```python
from build123d import *

# Parameters (mm, degrees)
BOSS_EXTRUDE1_DEPTH = 9
BOSS_EXTRUDE2_DEPTH = 11
SKETCH4_W           = 15
SKETCH4_H           = 5
CUT_EXTRUDE1_DEPTH  = 3


with BuildPart() as part:
    # Sketch2 → Boss-Extrude1 (new body)
    with BuildSketch(Plane(origin=(0, 0, 0), x_dir=(1, 0, 0), z_dir=(0, 1, 0))):
        with BuildLine():
            ThreePointArc((-13.134406493, 3.867125393), (0, 3), (13.134406493, 3.867125393))
            Line((13.134406493, 3.867125393), (13.134406493, -3.867125393))
            ThreePointArc((13.134406493, -3.867125393), (0, -3), (-13.134406493, -3.867125393))
            Line((-13.134406493, -3.867125393), (-13.134406493, 3.867125393))
        make_face()
    extrude(amount=BOSS_EXTRUDE1_DEPTH)

    # Sketch3 → Boss-Extrude2 (add)
    with BuildSketch(Plane(origin=(0, 9, 0), x_dir=(1, 0, 0), z_dir=(0, 1, 0))):
        with BuildLine():
            Line((13.134406493, -3.867125393), (13.134406493, 3.867125393))
            ThreePointArc((13.134406493, 3.867125393), (0, 3), (-13.134406493, 3.867125393))
            Line((-13.134406493, 3.867125393), (-13.134406493, -3.867125393))
            ThreePointArc((-13.134406493, -3.867125393), (0, -3), (13.134406493, -3.867125393))
        make_face()
    extrude(amount=BOSS_EXTRUDE2_DEPTH)

    # Sketch4 → Cut-Extrude1 (cut)
    with BuildSketch(Plane.XZ):
        Rectangle(SKETCH4_W, SKETCH4_H)
    extrude(amount=-CUT_EXTRUDE1_DEPTH, mode=Mode.SUBTRACT)


solid = part.part
```
Can you work these out from the model? Positions are in its coordinate system, mm. A direction names the side the tool comes from. Coordinates: 2 decimals unless noted, no trailing zeros. Loops run counter-clockwise (first coordinate to the right, second up) from the corner with the lowest first, then second, coordinate; pieces in that order, holes last. Notation, with made-up numbers: (82, -22) -> (93, -22) arc R16 ccw to (93, -5) -> close; hole circle Ø3 at (-25.75, 81). An arc over 180 degrees is marked (long way). Put each result on its own line as item: value. Start each with the question number.
Q1. Thinking about a two-plate mould opening in X: for faces 3 (the face through (13.134, 10, 0)), 4 (the face through (-13.134, 10, 0)), 5 (the face through (0, 20, 0)), 6 (the face through (0, 3, 0)), which applies, pulls with the +X half, pulls with the -X half, needs draft (parallel to the pull), parting line crosses it, or undercut?
Q2. I want a section at B-B (x = -4.5). Write out the boundary of the cut face in (y, z).
Q3. I want a section at D-D (x = -10.75). Write out the boundary of the cut face in (y, z), plus the area to 3 significant figures.
Q4. I'm going to push flat-ended pins straight in: P1, Ø3.5, axis at x = -3, y = 2, coming from the -Z side; P2, Ø6, axis at x = -9.5, y = 9.5, coming from the +Z side; P3, Ø2.5, axis at x = -1, y = 2, coming from the +Z side. Where does each tip first touch, or does it pass through?
Q5. I want a section at C-C (y = 13.25). Write out the boundary of the cut face in (x, z).
Q6. I want a section at A-A (z = -0.5). Write out the boundary of the cut face in (x, y).
Q7. If I drill on line 1 (Y direction, x = -5.75, z = 1.75); line 2 (X direction, y = 2.25, z = 0.5); line 3 (Z direction, x = 10, y = 8.5), over which ranges is the centre line in solid material (lowest first)? Write a range as [from, to].
Q8. For faces 1 (the face through (0, 10, -3)), 2 (the face through (7.5, 1, 0)), which set-ups out of +Z, -Z, +X, -X, +Y, -Y let a thin tool reach every point of the face, with its end or its side?
Taken from the geometry:
1. face 3: pulls with the +X half
1. face 4: pulls with the -X half
1. face 5: needs draft
1. face 6: undercut
2. outline: (0, -3.1) -> (20, -3.1) -> (20, 3.1) -> (0, 3.1) -> (0, 2.5) -> (3, 2.5) -> (3, -2.5) -> (0, -2.5) -> close
3. outline: (0, -3.58) -> (20, -3.58) -> (20, 3.58) -> (0, 3.58) -> close
3. area: 143 mm2
4. P1: stops at z = -3.11
4. P2: stops at z = 3.79
4. P3: stops at z = 3.03
5. outline: (-13.13, -3.87) arc R99.91 cw to (13.13, -3.87) -> (13.13, 3.87) arc R99.91 cw to (-13.13, 3.87) -> close
6. outline: (-13.13, 0) -> (-7.5, 0) -> (-7.5, 3) -> (7.5, 3) -> (7.5, 0) -> (13.13, 0) -> (13.13, 20) -> (-13.13, 20) -> close
7. line 1: y = [3, 20]
7. line 2: x = [-13.13, -7.5], [7.5, 13.13]
7. line 3: z = [-3.5, 3.5]
8. face 1: -Z, +Y, -Y
8. face 2: -Y
